Autodesk Inventor part; units mm, degrees
ref_plane "YZ Plane" through (0, 0, 0) normal (1, 0, 0) x (0, 1, 0)
ref_plane "XZ Plane" through (0, 0, 0) normal (0, 1, 0) x (-1, 0, 0)
ref_plane "XY Plane" through (0, 0, 0) normal (0, 0, 1) x (1, 0, 0)
sketch "Sketch1" plane through (0, 0, 0) normal (0, 0, 1) x (1, 0, 0)
  line L0 (111.125, 0) -> (104.775, 0)
  line L1 (6.35, 0) -> (0, 0)
  line L2 (0, 0) -> (0, -3.175)
  line L3 (0, -3.175) -> (-4.7752, -3.175)
  line L4 (-4.7752, -3.175) -> (-4.7752, -9.525)
  line L5 (-4.7752, -9.525) -> (0, -9.525)
  line L6 (0, -119.0625) -> (0, -107.9373)
  line L7 (0, -107.9373) -> (-4.7752, -107.9373)
  line L8 (-4.7752, -107.9373) -> (-4.7752, -101.5873)
  line L9 (-4.7752, -101.5873) -> (0, -101.5873)
  line L10 (0, -119.0625) -> (1.5875, -119.0625)
  line L11 (1.5875, -119.0625) -> (1.5875, -123.8377)
  line L12 (1.5875, -123.8377) -> (7.9375, -123.8377)
  line L13 (7.9375, -123.8377) -> (7.9375, -119.0625)
  line L14 (0, 0) -> (0, -3.175)
  line L15 (0, -9.525) -> (0, -101.5873)
  line L16 (0, -107.9373) -> (0, -119.0625)
  line L17 (0, -119.0625) -> (1.5875, -119.0625)
  line L18 (111.125, -3.175) -> (115.9002, -3.175)
  line L19 (115.9002, -3.175) -> (115.9002, -9.525)
  line L20 (115.9002, -9.525) -> (111.125, -9.525)
  line L21 (111.125, -3.175) -> (111.125, 0)
  line L22 (111.125, -107.9373) -> (115.9002, -107.9373)
  line L23 (115.9002, -107.9373) -> (115.9002, -101.5873)
  line L24 (115.9002, -101.5873) -> (111.125, -101.5873)
  line L25 (111.125, -119.0625) -> (111.125, -107.9373)
  line L26 (111.125, -101.5873) -> (111.125, -9.525)
  line L27 (111.125, -119.0625) -> (109.5375, -119.0625)
  line L28 (109.5375, -119.0625) -> (109.5375, -123.8377)
  line L29 (109.5375, -123.8377) -> (103.1875, -123.8377)
  line L30 (103.1875, -123.8377) -> (103.1875, -119.0625)
  line L31 (7.9375, -119.0625) -> (103.1875, -119.0625)
  line L32 (109.5375, -119.0625) -> (111.125, -119.0625)
  line L33 (6.35, -3.175) -> (3.175, -3.175)
  line L34 (3.175, -3.175) -> (3.175, -9.525)
  line L35 (3.175, -9.525) -> (6.35, -9.525)
  line L36 (6.35, -3.175) -> (6.35, 0)
  line L37 (104.775, -3.175) -> (107.95, -3.175)
  line L38 (107.95, -3.175) -> (107.95, -9.525)
  line L39 (107.95, -9.525) -> (104.775, -9.525)
  line L40 (104.775, 0) -> (104.775, -3.175)
  line L41 (6.35, -112.7125) -> (6.35, -100.0125)
  line L42 (6.35, -100.0125) -> (3.175, -100.0125)
  line L43 (3.175, -100.0125) -> (3.175, -93.6625)
  line L44 (3.175, -93.6625) -> (6.35, -93.6625)
  line L45 (6.35, -112.7125) -> (6.35, -100.0125)
  line L46 (6.35, -93.6625) -> (6.35, -9.525)
  line L47 (6.35, -112.7125) -> (7.9375, -112.7125)
  line L48 (7.9375, -112.7125) -> (7.9375, -115.8875)
  line L49 (7.9375, -115.8875) -> (14.2875, -115.8875)
  line L50 (14.2875, -115.8875) -> (14.2875, -112.7125)
  line L51 (7.9375, -112.7125) -> (6.35, -112.7125)
  line L52 (104.775, -112.7125) -> (103.1875, -112.7125)
  line L53 (103.1875, -112.7125) -> (103.1875, -115.8875)
  line L54 (103.1875, -115.8875) -> (96.8375, -115.8875)
  line L55 (96.8375, -115.8875) -> (96.8375, -112.7125)
  line L56 (104.775, -112.7125) -> (103.1875, -112.7125)
  line L57 (96.8375, -112.7125) -> (14.2875, -112.7125)
  line L58 (104.775, -112.7125) -> (104.775, -100.0125)
  line L59 (104.775, -100.0125) -> (107.95, -100.0125)
  line L60 (107.95, -100.0125) -> (107.95, -93.6625)
  line L61 (107.95, -93.6625) -> (104.775, -93.6625)
  line L62 (104.775, -9.525) -> (104.775, -93.6625)
  line L63 (104.775, -100.0125) -> (104.775, -112.7125)
  dimension "d0" = 119.0625
  dimension "d1" = 111.125
  dimension "d2" = 6.35
  dimension "d3" = 112.7125
  dimension "d4" = 98.425
  dimension "d7" = 119.0625
  dimension "d10" = 3.175
  dimension "d11" = 4.7752
  dimension "d12" = 6.35
  dimension "d13" = 11.1252
  dimension "d14" = 4.7752
  dimension "d15" = 6.35
  dimension "d16" = 1.5875
  dimension "d17" = 4.7752
  dimension "d18" = 6.35
  dimension "d19" = 4.7752
  dimension "d20" = 4.7752
  dimension "d21" = 1.5875
  dimension "d22" = 6.35
  dimension "d24" = 3.175
  dimension "d25" = 3.175
  dimension "d26" = 12.7
  dimension "d27" = 6.35
  dimension "d28" = 1.5875
  dimension "d29" = 3.175
  dimension "d30" = 6.35
  dimension "d31" = 1.5875
  dimension "d32" = 6.35
  dimension "d33" = 12.7
  dimension "d34" = 6.35
extrude "Extrusion1" add sketch "Sketch1" along normal blind 304.8
properties part number "CompactSlidePart2" material "Aluminum 6061"
Geometry check sheet. Reference: the model listing, model coordinates, mm. A direction names the side the tool comes from. Round coordinates to 2 decimals unless told otherwise and drop trailing zeros. Order: outer loops, then holes, each group sorted by start corner. A loop starts at its lowest first (then second) coordinate and runs counter-clockwise, first axis right, second up. Notation, with made-up numbers: (5.5, -21) - (13.5, -21) arc R31 cw to (13.5, 5) - close; hole circle Ø7 at (8, -24.5). An arc over 180 degrees is marked (long way). One line per question, with ' | ' between items. Start each with the question number.
(1) Depth check by flat-ended pin: pin 1 Ø1.7 at (x, z) = (110.5, 213.5) entering from -Y; pin 2 Ø2.5 at (y, z) = (-121.5, 203) entering from -X; pin 3 Ø6 at (x, z) = (100, 104.5) entering from +Y; pin 4 Ø5 at (x, y) = (10.5, -71.5) entering from +Z. Enter the tip coordinate at first touch or a pass-through.
(2) Sectioned sample at B-B on x = 85.5. Record the cut outline in (y, z).
(3) Sectioned sample at A-A on y = -26.5. Record the cut outline in (x, z) (3 decimals).
(4) Access from +Z, -Z, +X, -X, +Y, -Y to the whole of each face (thin tool, end or side, straight path). Record for faces 5 (the flat face through (111.125, -56, 150)), 6 (the flat face through (6.35, -106, 150)), 7 (the flat face through (111.125, -114, 150)), 8 (the flat face through (107.95, -97, 150)), 9 (the flat face through (0, -55, 150)).
(5) Thickness scan on L1, parallel to X at y = -36.5, z = 29.5 (3 decimals); L2, parallel to Y at x = 4, z = 132 (1 decimal); L3, parallel to Y at x = 15.5, z = 283. Record the ranges inside material, lowest first. Write a range as [from, to].
(6) Release check for a two-part mould opening along X. For faces 1 (the flat face through (56, -112.712, 150)), 2 (the flat face through (11, -115.888, 150)), 3 (the flat face through (115.9, -105, 150)), 4 (the flat face through (-4.775, -6, 150)) record: released by +X, released by -X, zero draft, split by the parting line, or undercut.
Conclusion:
1) pin 1: stops at y = -119.06 | pin 2: stops at x = 1.59 | pin 3: stops at y = -115.89 | pin 4: passes through
2) outline: (-119.06, 0) - (-112.71, 0) - (-112.71, 304.8) - (-119.06, 304.8) - close
3) outline: (0, 0) - (6.35, 0) - (6.35, 304.8) - (0, 304.8) - close; (104.775, 0) - (111.125, 0) - (111.125, 304.8) - (104.775, 304.8) - close
4) face 5: +Z, -Z, +X | face 6: +Z, -Z, +Y | face 7: +Z, -Z, +X, -Y | face 8: +Z, -Z | face 9: +Z, -Z, -X
5) L1: x = [0, 6.35], [104.775, 111.125] | L2: y = [-123.8, -100], [-93.7, -9.5], [-3.2, 0] | L3: y = [-119.06, -112.71]
6) face 1: undercut | face 2: undercut | face 3: released by +X | face 4: released by -X
